from build123d import *

# Parameters (mm, degrees)
ESBO_O1_W                = 38.4
ESBO_O1_H                = 8.4
RESSALTO_EXTRUS_O1_DEPTH = 2.4
ESBO_O2_W                = 1.6
ESBO_O2_H                = 1.6
CORTE_EXTRUS_O1_DEPTH    = 2.5
PADR_O_LINEAR1_COUNT     = 16
PADR_O_LINEAR1_PITCH     = 2.56
ESBO_O3_R                = 0.51
CORTE_EXTRUS_O2_DEPTH    = 21.228939666
PADR_O_LINEAR2_COUNT     = 15
PADR_O_LINEAR2_PITCH     = 2.543
ESBO_O6_W                = 18.080220827
ESBO_O6_H                = 8.4
CORTE_EXTRUS_O3_DEPTH    = 10


with BuildPart() as part:
    # Esboço1 → Ressalto-extrusão1 (new body)
    with BuildSketch(Plane.XY):
        Rectangle(ESBO_O1_W, ESBO_O1_H)
    extrude(amount=RESSALTO_EXTRUS_O1_DEPTH)

    # Esboço2 → Corte-extrusão1 (cut)
    with BuildSketch(Plane(origin=(0, 4.2, 0), x_dir=(1, 0, 0), z_dir=(0, 1, 0))):
        with Locations((-18, -1.2)):
            Rectangle(ESBO_O2_W, ESBO_O2_H)
    corte_extrus_o1 = extrude(amount=-CORTE_EXTRUS_O1_DEPTH, mode=Mode.SUBTRACT)

    # Padrão linear1: Corte-extrusão1 ×16
    with Locations(*[(i * PADR_O_LINEAR1_PITCH, 0, 0) for i in range(1, PADR_O_LINEAR1_COUNT)]):
        add(corte_extrus_o1, mode=Mode.SUBTRACT)

    # Esboço3 → Corte-extrusão2 (cut, through all)
    with BuildSketch(Plane(origin=(0, 1.7, 0), x_dir=(1, 0, 0), z_dir=(0, 1, 0))):
        with Locations(Location((-18, -1.2, 0), (0, 0, 270))):
            Circle(ESBO_O3_R)
    corte_extrus_o2 = extrude(amount=-CORTE_EXTRUS_O2_DEPTH, mode=Mode.SUBTRACT)

    # Padrão linear2: Corte-extrusão2 ×15
    with Locations(*[(i * PADR_O_LINEAR2_PITCH, 0, 0) for i in range(1, PADR_O_LINEAR2_COUNT)]):
        add(corte_extrus_o2, mode=Mode.SUBTRACT)

    # Esboço6 → Corte-extrusão3 (cut)
    with BuildSketch(Plane.XY.offset(2.4)):
        with Locations((10.159889587, 0)):
            Rectangle(ESBO_O6_W, ESBO_O6_H)
    extrude(amount=-CORTE_EXTRUS_O3_DEPTH, mode=Mode.SUBTRACT)


solid = part.part
The model under review builds one solid part; all positions refer to its coordinate system, in mm. A direction names the side the tool comes from. Round coordinates to 2 decimals unless told otherwise and drop trailing zeros. Write each loop counter-clockwise with the first axis right and the second up, starting at its lowest first coordinate (ties: lowest second). Pieces come first, ordered by that corner, then holes. Notation, with made-up numbers: (-25, 41.5) - (-5, 41.5) arc R8 cw to (-5, 48.5) - close; hole circle Ø2 at (34.25, 74). An arc over 180 degrees is marked (long way). One line per item, written item: value. Start each with the question number.
1. Consider section B-B on z = 1.2. State how many separate pieces and enclosed holes the cut face has, and give its area (3 significant figures).
2. To check wall thickness, follow L1, parallel to Z at x = -14.75, y = 3.25; L2, parallel to Z at x = -5.5, y = -2.75; L3, parallel to Y at x = -5, z = 0.5. State the ranges of each line that lie inside material, in increasing order. Write a range as from..to.
3. The part is to be moulded in two halves that separate along Z. For faces 1 (the face through (-17.2, 3, 1)), 2 (the face through (-9, 0, 0)), 3 (the face through (-9, -4.2, 1)), 4 (the face through (-18, 3, 0.4)), say which applies: released by +Z, released by -Z, zero draft, split by the parting line, or undercut.
4. Machinability: for faces 5 (the face through (-8.56, 3, 1)), 6 (the face through (-2.4, -1.21, 0.82)), which of the approach directions +Z, -Z, +X, -X, +Y, -Y give a long, thin tool a straight path to every point of the face, cutting with its end or side? Answer none if there is none.
5. Clearance check with a flat-ended pin moving along its axis: P1, Ø0.8, axis at x = -10.5, z = 1.5, coming from the +Y side. State where the tip first meets the part, or that it passes through.
6. Consider section A-A on x = -18. Write out the cut boundary in (y, z).
Checks:
1. separate pieces: 9
1. enclosed holes: 0
1. area: 90.5 mm^2
2. L1: z = 0..0.4, 2..2.4
2. L2: z = 0..0.74, 1.66..2.4
2. L3: y = -4.2..1.7
3. face 1: undercut
3. face 2: released by -Z
3. face 3: zero draft
3. face 4: undercut
4. face 5: +Y
4. face 6: +Y, -Y
5. P1: stops at y = 1.7
6. outline: (-4.2, 0) - (4.2, 0) - (4.2, 0.4) - (1.7, 0.4) - (1.7, 0.69) - (-4.2, 0.69) - close; (-4.2, 1.71) - (1.7, 1.71) - (1.7, 2) - (4.2, 2) - (4.2, 2.4) - (-4.2, 2.4) - close
